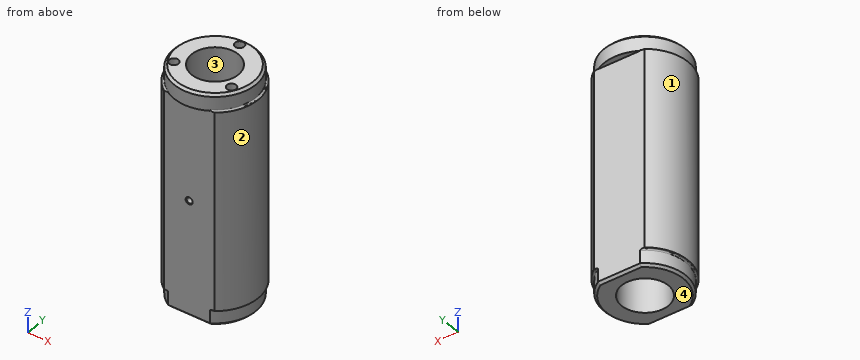
from build123d import *

# Parameters (mm, degrees)
BOSS_EXTRUDE1_DEPTH         = 49.5
BOSS_EXTRUDE1_DEPTH_BACK    = 49.5
BOSS_EXTRUDE2_DEPTH         = 42.5
BOSS_EXTRUDE2_DEPTH_BACK    = 42.5
BOSS_EXTRUDE3_START         = -7
BOSS_EXTRUDE3_DEPTH         = 7
SKETCH6_R                   = 2
SKETCH6_R_2                 = 2.0000000000012577
SKETCH6_R_3                 = 2.0000000000018354
CUT_EXTRUDE1_DEPTH          = 5
M3_TAPPED_HOLE1_D           = 2.5
M3_TAPPED_HOLE1_DEPTH       = 7.5
M3_TAPPED_HOLE1_CSINK_D     = 3.05
M3_TAPPED_HOLE1_CSINK_ANGLE = 90
M3_TAPPED_HOLE1_TIP         = 0.7510757737844503
FILLET1_R                   = 0.5
CHAMFER1_SIZE               = 1
CHAMFER2_SIZE               = 1


with BuildPart() as part:
    # Sketch1 → Boss-Extrude1 (new, two sides: drawn at the far end of the back side and taken through both)
    with BuildSketch(Plane.XY.offset(-BOSS_EXTRUDE1_DEPTH_BACK)):
        with BuildLine():
            Line((9.013878188660517, 15), (0, 15))
            Line((0, 15), (0, 10.000000000000004))
            ThreePointArc((-4.824e-14, 10.000000000000004), (7.07106781186546, 7.071067811865495), (10.000000000000004, 0))
            ThreePointArc((10.000000000000004, -2.45e-15), (7.071067811865457, -7.071067811865499), (-5.513e-14, -10.000000000000004))
            Line((0, -10.000000000000007), (0, -15))
            Line((0, -14.999999999999998), (9.013878188660513, -14.999999999999996))
            ThreePointArc((9.013878188660447, -14.999999999999721), (15.231429156542696, -8.617050878880846), (17.500000000000004, -4.29e-15))
            ThreePointArc((17.500000000000004, 0), (15.231429156542696, 8.617050878880846), (9.013878188660442, 14.999999999999723))
        make_face()
        with BuildLine():
            Line((0, 10.000000000000004), (0, 15))
            Line((0, 15), (-9.013878188659975, 15))
            ThreePointArc((-9.013878188659975, 15.000000000000002), (-17.500000000000004, 1.769e-14), (-9.01387818866, -14.99999999999999))
            Line((-9.013878188659985, -15), (0, -14.999999999999998))
            Line((0, -15), (0, -10.000000000000007))
            ThreePointArc((-5.513e-14, -10.000000000000004), (-10.000000000000004, 1.22e-15), (-4.824e-14, 10.000000000000004))
        make_face()
    extrude(amount=BOSS_EXTRUDE1_DEPTH + BOSS_EXTRUDE1_DEPTH_BACK)

    # Sketch1<23> → Boss-Extrude2 (add, two sides: drawn at the far end of the back side and taken through both)
    with BuildSketch(Plane.XY.offset(-BOSS_EXTRUDE2_DEPTH_BACK)):
        with BuildLine():
            Line((-9.013878188659975, 15), (-10.828203913853855, 15))
            ThreePointArc((-10.828203913853855, 15.000000000000004), (-18.5, -5.95e-15), (-10.828203913853852, -15.000000000000005))
            Line((-10.828203913853855, -15), (-9.013878188659985, -15))
            ThreePointArc((-9.01387818866, -14.99999999999999), (-17.500000000000004, 1.769e-14), (-9.013878188659975, 15.000000000000002))
        make_face()
        with BuildLine():
            ThreePointArc((18.5, 0), (16.470758519362374, 8.424020049646833), (10.828203913853855, 15))
            Line((10.828203913853855, 15), (9.013878188660517, 15))
            ThreePointArc((9.013878188660442, 14.999999999999723), (15.231429156542696, 8.617050878880846), (17.500000000000004, 0))
            ThreePointArc((17.500000000000004, -4.29e-15), (15.231429156542696, -8.617050878880846), (9.013878188660447, -14.999999999999721))
            Line((9.013878188660513, -14.999999999999996), (10.828203913853855, -14.999999999999996))
            ThreePointArc((10.828203913853848, -15.000000000000009), (16.47075851936237, -8.42402004964684), (18.5, -4.53e-15))
        make_face()
    extrude(amount=BOSS_EXTRUDE2_DEPTH + BOSS_EXTRUDE2_DEPTH_BACK)

    # Sketch5 → Boss-Extrude3 (add)
    with BuildSketch(Plane.XY.offset(49.5).offset(BOSS_EXTRUDE3_START)):
        with BuildLine():
            ThreePointArc((9.013878188660444, 14.999999999999721), (2.7267e-13, 17.500000000000004), (-9.013878188659977, 15.000000000000002))
            Line((-9.013878188659975, 15), (9.013878188660518, 14.99999999999984))
        make_face()
        with BuildLine():
            ThreePointArc((-9.013878188659985, -14.999999999999998), (2.6645e-13, -17.500000000000007), (9.01387818866044, -14.999999999999726))
            Line((9.013878188660513, -14.999999999999838), (-9.013878188659987, -14.999999999999998))
        make_face()
    extrude(amount=BOSS_EXTRUDE3_DEPTH)

    # Sketch6 → Cut-Extrude1 (cut)
    with BuildSketch(Plane.XY.offset(49.5)):
        with Locations((0, 14.25)):
            Circle(SKETCH6_R)
        with Locations((12.340862003929768, -7.124999999999125)):
            Circle(SKETCH6_R_2)
        with Locations((-12.340862003926736, -7.12500000000088)):
            Circle(SKETCH6_R_3)
    extrude(amount=-CUT_EXTRUDE1_DEPTH, mode=Mode.SUBTRACT)

    # M3 Tapped Hole1
    with Locations(Plane(origin=(2.4e-15, -14.999999999999998, 0), x_dir=(-1, -1.6e-16, 0), z_dir=(1.6e-16, -1, 0))):
        with Locations((0, 0)):
            CounterSinkHole(M3_TAPPED_HOLE1_D / 2, M3_TAPPED_HOLE1_CSINK_D / 2, depth=M3_TAPPED_HOLE1_DEPTH, counter_sink_angle=M3_TAPPED_HOLE1_CSINK_ANGLE)
            with Locations((0, 0, -(M3_TAPPED_HOLE1_DEPTH + M3_TAPPED_HOLE1_TIP / 2))):  # 118° drill point
                Cone(0, M3_TAPPED_HOLE1_D / 2, M3_TAPPED_HOLE1_TIP, mode=Mode.SUBTRACT)

    # Fillet1
    # the kernel refuses this fillet: 0.5 mm, written as the material it adds along each edge
    with BuildSketch(Plane(origin=(-1.421e-14, 5.77e-15, 42.5), x_dir=(0.45254890557349203, -0.8917395853410538, 0), z_dir=(-0.8917395853410538, -0.45254890557349203, 0))) as fillet1_piece_1_section:
        with BuildLine():
            CenterArc((17.500000000000018 + FILLET1_R, FILLET1_R), FILLET1_R, 180, 90)
            Line((17.500000000000018 + FILLET1_R, 0), (17.500000000000018, 0))
            Line((17.500000000000018, 0), (17.500000000000018, FILLET1_R))
        make_face()
    fillet1_piece_1 = revolve(axis=Axis((-1.421e-14, 5.77e-15, 42.5), (0, 0, 1)), revolution_arc=126.18532587010755, mode=Mode.PRIVATE)
    fillet1_piece_1 = split(fillet1_piece_1, bisect_by=Plane(origin=(17.637648609148254, 15, 42.63764860914824), z_dir=(0, -1, 0)), keep=Keep.TOP, mode=Mode.PRIVATE)
    fillet1_piece_1 = split(fillet1_piece_1, bisect_by=Plane(origin=(17.637648609148258, -14.999999999999995, 42.63764860914824), z_dir=(-2e-16, 1, 0)), keep=Keep.TOP, mode=Mode.PRIVATE)
    add(fillet1_piece_1)
    with BuildSketch(Plane(origin=(-1.066e-14, -6.22e-15, -42.5), x_dir=(0.4525489055734917, 0.891739585341054, 0), z_dir=(-0.891739585341054, 0.4525489055734917, 0))) as fillet1_piece_2_section:
        with BuildLine():
            CenterArc((17.50000000000003 + FILLET1_R, FILLET1_R), FILLET1_R, 180, 90)
            Line((17.50000000000003 + FILLET1_R, 0), (17.50000000000003, 0))
            Line((17.50000000000003, 0), (17.50000000000003, FILLET1_R))
        make_face()
    fillet1_piece_2 = revolve(axis=Axis((-1.066e-14, -6.22e-15, -42.5), (0, 0, -1)), revolution_arc=126.18532587010758, mode=Mode.PRIVATE)
    fillet1_piece_2 = split(fillet1_piece_2, bisect_by=Plane(origin=(17.63764860914827, 15, -42.63764860914825), z_dir=(0, -1, 0)), keep=Keep.TOP, mode=Mode.PRIVATE)
    fillet1_piece_2 = split(fillet1_piece_2, bisect_by=Plane(origin=(17.637648609148272, -14.999999999999995, -42.63764860914825), z_dir=(-2e-16, 1, 0)), keep=Keep.TOP, mode=Mode.PRIVATE)
    add(fillet1_piece_2)
    with BuildSketch(Plane(origin=(1.78e-15, -1.33e-15, 42.5), x_dir=(-0.4525489055734672, -0.8917395853410666, 0), z_dir=(0.8917395853410666, -0.4525489055734672, 0))) as fillet1_piece_3_section:
        with BuildLine():
            CenterArc((17.50000000000002 + FILLET1_R, -FILLET1_R), FILLET1_R, 90, 90)
            Line((17.50000000000002 + FILLET1_R, 0), (17.50000000000002, 0))
            Line((17.50000000000002, 0), (17.50000000000002, -FILLET1_R))
        make_face()
    fillet1_piece_3 = revolve(axis=Axis((1.78e-15, -1.33e-15, 42.5), (0, 0, -1)), revolution_arc=126.18532587011086, mode=Mode.PRIVATE)
    fillet1_piece_3 = split(fillet1_piece_3, bisect_by=Plane(origin=(-17.637648609148275, 15, 42.63764860914824), z_dir=(0, -1, 0)), keep=Keep.TOP, mode=Mode.PRIVATE)
    fillet1_piece_3 = split(fillet1_piece_3, bisect_by=Plane(origin=(-17.637648609148272, -15.000000000000002, 42.63764860914824), z_dir=(-2e-16, 1, 0)), keep=Keep.TOP, mode=Mode.PRIVATE)
    add(fillet1_piece_3)
    with BuildSketch(Plane(origin=(1.78e-15, -1.33e-15, -42.5), x_dir=(-0.4525489055734672, -0.8917395853410666, 0), z_dir=(0.8917395853410666, -0.4525489055734672, 0))) as fillet1_piece_4_section:
        with BuildLine():
            CenterArc((17.500000000000007 + FILLET1_R, FILLET1_R), FILLET1_R, 180, 90)
            Line((17.50000000000001, FILLET1_R), (17.500000000000007, 0))
            Line((17.500000000000007, 0), (17.500000000000007 + FILLET1_R, 0))
        make_face()
    fillet1_piece_4 = revolve(axis=Axis((1.78e-15, -1.33e-15, -42.5), (0, 0, -1)), revolution_arc=126.18532587011086, mode=Mode.PRIVATE)
    fillet1_piece_4 = split(fillet1_piece_4, bisect_by=Plane(origin=(-17.637648609147508, 15, -42.6376486091475), z_dir=(0, -1, 0)), keep=Keep.TOP, mode=Mode.PRIVATE)
    fillet1_piece_4 = split(fillet1_piece_4, bisect_by=Plane(origin=(-17.637648609147504, -15.000000000000002, -42.6376486091475), z_dir=(-2e-16, 1, 0)), keep=Keep.TOP, mode=Mode.PRIVATE)
    add(fillet1_piece_4)

    # Chamfer1
    chamfer1_edges = [part.edges().sort_by_distance(p)[0] for p in [
        (9.01387818866, 14.99999999999999, 49.5),
        (-17.500000000000007, 1.066e-14, -49.5),
        (17.500000000000004, 5.77e-15, -49.5),
    ]]
    chamfer(chamfer1_edges, length=CHAMFER1_SIZE)

    # Chamfer2
    chamfer2_edges = [part.edges().sort_by_distance(p)[0] for p in [
        (1.78e-15, -14.999999999999927, -49.5),
        (1.421e-14, 14.999999999999932, -49.5),
    ]]
    chamfer(chamfer2_edges, length=CHAMFER2_SIZE)


solid = part.part
Geometry: final body of the model. Coordinates: model frame, mm. Face numbers are marked on the shaded views. Give positions to 0.01 mm unless a question says otherwise; leave off trailing zeros. Write each loop counter-clockwise with the first axis right and the second up, starting at its lowest first coordinate (ties: lowest second). Pieces come first, ordered by that corner, then holes.
(1) Cut plane C-C, the plane z = -20. Return loops of the section in (x, y), then the cut area to 3 significant figures.
(2) Ray query, line 1 (Y direction, x = -1, z = 10); line 2 (Y direction, x = 0.5, z = -37); line 3 (Z direction, x = 0, y = -12.1). Return the intervals inside material, ascending.
(3) Cut plane A-A, the plane x = 0. Return loops of the section in (y, z) (3 decimals), then the cut area to 3 significant figures.
(4) Mould query, pull axis X, two halves, no side actions, for the marked faces 1, 2, 3 and 4. Classes: released by +X, released by -X, zero draft, split by the parting line, or undercut.
(5) Cut plane B-B, the plane z = 0. Return loops of the section in (x, y) (3 decimals), then the cut area to 3 significant figures.
(6) First-contact query: P1, Ø2, axis at x = 0, z = 0, coming from the -Y side; P2, Ø10, axis at x = 0, z = -17, coming from the +Y side; P3, Ø10, axis at x = -4.5, z = -13, coming from the -Y side. Flat tips, straight axial feed; report the tip coordinate or a pass-through.
Values follow:
1. outline: (-10.83, -15) - (10.83, -15) arc R18.5 ccw to (10.83, 15) - (-10.83, 15) arc R18.5 ccw to start; hole circle Ø20 at (0, 0)
1. area: 658 mm2
2. line 1: y = -15 to -9.95, 9.95 to 15
2. line 2: y = -15 to -9.99, 9.99 to 15
2. line 3: z = -49.5 to -1.25, 1.25 to 49.5
3. outline: (-17.5, 42.5) - (-15, 42.5) - (-15, 1.525) - (-14.725, 1.25) - (-10, 1.25) - (-10, 49.5) - (-16.5, 49.5) - (-17.5, 48.5) - close; (-15, -48.5) - (-14, -49.5) - (-10, -49.5) - (-10, -1.25) - (-14.725, -1.25) - (-15, -1.525) - close; (10, -49.5) - (14, -49.5) - (15, -48.5) - (15, 42.5) - (17.5, 42.5) - (17.5, 48.5) - (16.5, 49.5) - (16.25, 49.5) - (16.25, 44.5) - (12.25, 44.5) - (12.25, 49.5) - (10, 49.5) - close
3. area: 990 mm2
4. face 1: released by -X
4. face 2: released by +X
4. face 3: undercut
4. face 4: zero draft
5. outline: (-10.828, -15) - (-1.525, -15) - (-1.25, -14.725) - (-1.25, -9.922) arc R10 cw (long way) to (1.25, -9.922) - (1.25, -14.725) - (1.525, -15) - (10.828, -15) arc R18.5 ccw to (10.828, 15) - (-10.828, 15) arc R18.5 ccw to start
5. area: 645 mm2
6. P1: stops at y = 9.95
6. P2: stops at y = 15
6. P3: stops at y = -15
